Autodesk Inventor part; units mm, degrees
ref_plane "YZ Plane" through (0, 0, 0) normal (1, 0, 0) x (0, 1, 0)
ref_plane "XZ Plane" through (0, 0, 0) normal (0, 1, 0) x (-1, 0, 0)
ref_plane "XY Plane" through (0, 0, 0) normal (0, 0, 1) x (1, 0, 0)
sketch "Sketch2" plane through (0, 0, 0) normal (0, 0, 1) x (1, 0, 0)
  line L0 (0, 0) -> (107.95, 0)
  line L1 (107.95, 0) -> (107.95, 25.4)
  line L2 (0, 25.4) -> (0, 0)
  arc A0 (75.2475, 25.4) -> (102.5525, 25.4) centre (88.9, 25.4) ccw
  line L3 (107.95, 25.4) -> (102.5525, 25.4)
  line L4 (75.2475, 25.4) -> (0, 25.4)
  dimension "d0" = 107.95
  dimension "d1" = 25.4
  dimension "d2" = 27.305
  dimension "d3" = 88.9
extrude "Extrusion1" add sketch "Sketch2" along normal mid plane 6.35
sketch "Sketch3" plane through (0, 0, 0) normal (0, 0, 1) x (1, 0, 0)
  line L0 (0, 0) -> (0, 25.4)
  line L1 (0, 25.4) -> (75.2475, 25.4)
  line L2 (107.95, 0) -> (0, 0)
  line L3 (0, 25.4) -> (6.35, 25.4)
  line L4 (6.35, 25.4) -> (6.35, 0)
  line L5 (6.35, 0) -> (0, 0)
  line L6 (0, 0) -> (0, 25.4)
  dimension "d17" = 6.35
extrude "Extrusion2" add sketch "Sketch3" along normal mid plane 44.45
sketch "Sketch4" plane through (6.35, 0, 3.175) normal (1, 0, 0) x (0, 0, -1)
  line L0 (-19.05, 0) -> (-19.05, 25.4)
  line L1 (-19.05, 25.4) -> (0, 25.4)
  line L2 (0, 0) -> (-19.05, 0)
  line L3 (0, 25.4) -> (0, 0)
  line L4 (-19.05, 25.4) -> (25.4, 25.4) construction
  line L5 (-9.525, 25.4) -> (-9.525, 0) construction
  point P0 (3.175, 0)
  point P1 (-9.525, 19.05)
  point P2 (-9.525, 6.35)
  dimension "d8" = 6.35
  dimension "d9" = 6.35
hole "Hole1" at (6.35, 19.05, 12.7) at (6.35, 6.35, 12.7) direction (-1, 0, 0) diameter 4.4958 end through all
mirror "Mirror1" about plane through (0, 0, 0) normal (0, 0, 1) of "Hole1"
ref_plane "Work Plane1" through (0, 0, 0) normal (0, 0, 1) x (1, 0, 0)
equation "\"d0\" = supportLength"
equation "\"d1\" = supportHeight"
equation "\"d2\" = pipeDiameter"
equation "\"d3\" = distanceFromWallToPipeCenter"
equation "\"d4\" = supportWidth"
equation "\"d17\" = screwHoldDepth"
equation "\"d6\" = totalScrewHoldWidth"
equation "\"pipeDiameter\" = 27.305"
equation "\"distanceFromWallToPipeCenter\" = 88.9"
equation "\"supportLength\" = 107.95"
equation "\"supportHeight\" = 25.4"
equation "\"supportWidth\" = 6.35"
equation "\"screwHoldDepth\" = 6.35"
equation "\"screwHoldWidthExtension\" = 19.05"
equation "\"totalScrewHoldWidth\" = supportWidth + 2 * screwHoldWidthExtension"
equation "\"screwPositionFromTop\" = 6.35"
properties part number "irrigationPipeSupport"
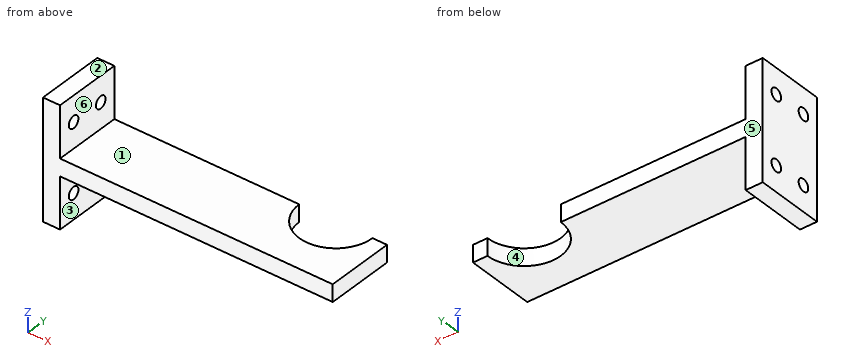
For this review, take the finished solid that the model builds, in its own axes (mm). Face numbers are marked on the shaded views. A direction names the side the tool comes from. Coordinates: 2 decimals unless noted, no trailing zeros. Order: outer loops, then holes, each group sorted by start corner. A loop starts at its lowest first (then second) coordinate and runs counter-clockwise, first axis right, second up. Notation, with made-up numbers: (22.5, 4) - (42.5, 4) arc R37 ccw to (42.5, 42) - close; hole circle Ø6 at (-5.75, 70). An arc over 180 degrees is marked (long way). Answer as a JSON object with one key per item and string values. Group by question number.
1. For the marked faces 1, 2 and 3, list the 3-axis set-ups (+Z, -Z, +X, -X, +Y, -Y) from which the entire face can be reached by the end or side of a thin tool; tool diameter is ignored.
2. We need section A-A on y = 6.35. State the section outline as (x, z) points (3 decimals), then the cut area to 3 significant figures.
3. We need section B-B on z = -12.7. State the section outline as (x, y) points.
4. We need section D-D on x = 88.9. State the section outline as (y, z) points (1 decimal).
5. Clearance check with a flat-ended pin moving along its axis: P1, Ø7, axis at y = 6.35, z = -12.7, coming from the +X side. State where the tip first meets the part, or that it passes through.
6. We need section C-C on y = 15. State the section outline as (x, z) points (3 decimals), then the cut area to 3 significant figures.
7. For probe 1 along Y at (x, z) = (4.25, -12.7); probe 2 along Z at (x, y) = (2, 6.35) (3 decimals); probe 3 along Y at (x, z) = (4, -12), list the stretches that pass through material, from the lowest coordinate up.
8. The part is to be moulded in two halves that separate along X. For the marked faces 4, 5 and 6, say which applies: pulls with the +X half, pulls with the -X half, needs draft (parallel to the pull), parting line crosses it, or undercut.
Final values:
{
 "1": {"face 1": "+Z, +X, +Y, -Y", "face 2": "+Z, +X, -X, +Y, -Y", "face 3": "-Z, +X, +Y, -Y"},
 "2": {"outline": "(0, -22.225) - (6.35, -22.225) - (6.35, -14.948) - (0, -14.948) - close; (0, -10.452) - (6.35, -10.452) - (6.35, -3.175) - (107.95, -3.175) - (107.95, 3.175) - (6.35, 3.175) - (6.35, 10.452) - (0, 10.452) - close; (0, 14.948) - (6.35, 14.948) - (6.35, 22.225) - (0, 22.225) - close", "area": "870 mm²"},
 "3": {"outline": "(0, 0) - (6.35, 0) - (6.35, 4.1) - (0, 4.1) - close; (0, 8.6) - (6.35, 8.6) - (6.35, 16.8) - (0, 16.8) - close; (0, 21.3) - (6.35, 21.3) - (6.35, 25.4) - (0, 25.4) - close"},
 "4": {"outline": "(0, -3.2) - (11.7, -3.2) - (11.7, 3.2) - (0, 3.2) - close"},
 "5": {"P1": "x = 6.35"},
 "6": {"outline": "(0, -22.225) - (6.35, -22.225) - (6.35, -3.175) - (80.055, -3.175) - (80.055, 3.175) - (6.35, 3.175) - (6.35, 22.225) - (0, 22.225) - close; (97.745, -3.175) - (107.95, -3.175) - (107.95, 3.175) - (97.745, 3.175) - close", "area": "815 mm²"},
 "7": {"probe 1": "0 to 4.1, 8.6 to 16.8, 21.3 to 25.4", "probe 2": "-22.225 to -14.948, -10.452 to 10.452, 14.948 to 22.225", "probe 3": "0 to 4.21, 8.49 to 16.91, 21.19 to 25.4"},
 "8": {"face 4": "undercut", "face 5": "needs draft", "face 6": "pulls with the +X half"}
}
